Here's how the part is built. I have some questions about the finished solid (model axes, mm). A direction names the side the tool comes from. Round coordinates to 2 decimals unless told otherwise and drop trailing zeros. Write each loop counter-clockwise with the first axis right and the second up, starting at its lowest first coordinate (ties: lowest second). Pieces come first, ordered by that corner, then holes. Notation, with made-up numbers: (-14, 15) -> (27, 15) arc R19 ccw to (27, 21) -> close; hole circle Ø11 at (9, 87.5). An arc over 180 degrees is marked (long way). Answer in a Markdown table with one row per item. Add a question column.
from build123d import *

# Parameters (mm, degrees)
BOSS_EXTRUDE1_DEPTH = 2


with BuildPart() as part:
    # Sketch3 → Boss-Extrude1 (new body)
    with BuildSketch(Plane(origin=(0, 0, 0), x_dir=(0, 0, -1), z_dir=(1, 0, 0))):
        with BuildLine():
            Line((-58.824606693, -2534.80652233), (-1.666930044, -2633.80652233))
            ThreePointArc((-1.666930044, -2633.80652233), (15.902289338, -2651.375741711), (39.902289338, -2657.80652233))
            Line((39.902289338, -2657.80652233), (202.448497275, -2657.80652233))
            ThreePointArc((202.448497275, -2657.80652233), (226.448497275, -2651.375741711), (244.017716657, -2633.80652233))
            Line((244.017716657, -2633.80652233), (301.175393307, -2534.80652233))
            Line((301.175393307, -2534.80652233), (240.287893307, -2534.80652233))
            Line((240.287893307, -2534.80652233), (240.287893307, -2532.80652233))
            Line((240.287893307, -2532.80652233), (216.287893307, -2532.80652233))
            Line((216.287893307, -2532.80652233), (216.287893307, -2534.80652233))
            Line((216.287893307, -2534.80652233), (155.400393307, -2534.80652233))
            Line((155.400393307, -2534.80652233), (155.400393307, -2572.30652233))
            ThreePointArc((155.400393307, -2572.30652233), (153.643033994, -2576.549163017), (149.400393307, -2578.30652233))
            Line((149.400393307, -2578.30652233), (92.950393307, -2578.30652233))
            ThreePointArc((92.950393307, -2578.30652233), (88.70775262, -2576.549163017), (86.950393307, -2572.30652233))
            Line((86.950393307, -2572.30652233), (86.950393307, -2534.80652233))
            Line((86.950393307, -2534.80652233), (43.175393307, -2534.80652233))
            Line((43.175393307, -2534.80652233), (43.175393307, -2532.80652233))
            Line((43.175393307, -2532.80652233), (19.175393307, -2532.80652233))
            Line((19.175393307, -2532.80652233), (19.175393307, -2534.80652233))
            Line((19.175393307, -2534.80652233), (-58.824606693, -2534.80652233))
        make_face()
    extrude(amount=BOSS_EXTRUDE1_DEPTH)


solid = part.part
Item 1: If we section it at C-C on z = -127: Please give me the cut outline in (x, y), then the cut area to 3 significant figures.
Item 2: If we mould it in two halves opening along Z, with no side actions, what happens to faces 3 (the flat face through (0.99, -2583.61, 30.65)), 4 (the cylindrical face through (0.99, -2576.5, -153.69)), 5 (the cylindrical face through (0.986, -2651.551, -226.143))? For each: pulls with the +Z half, pulls with the -Z half, needs draft (parallel to the pull), parting line crosses it, or undercut.
Item 3: I need wall thicknesses on line 1 along Y through (x, z) = (0.7, -187.5); line 2 along Z through (x, y) = (0.9, -2557.5); line 3 along Y through (x, z) = (0.6, -125). Which ranges of each line are inside material? Lowest first, please. Write a range as from..to.
Item 4: If we section it at B-B on x = 1.4: Please give me the cut outline in (y, z), then the cut area to 3 significant figures.
Item 5: If we section it at A-A on y = -2548.5: Please give me the cut outline in (x, z), then the cut area to 3 significant figures.
Item 6: For P1, Ø0.6, axis at x = 1, y = -2533.5, coming from the -Z side; P2, Ø0.6, axis at x = 1, y = -2560, coming from the -Z side; P3, Ø1, axis at x = 0.5, z = -101.5, coming from the +Y side, each with a flat end and sliding along its axis, tell me the tip position at first contact or that it passes through.
Item 7: If we section it at D-D on y = -2596.5: Please give me the cut outline in (x, z).
Item 8: On a 3-axis mill with a long thin cutter (end or side, diameter ignored), from which of +Z, -Z, +X, -X, +Y, -Y can I reach the whole of each face in a straight line? I mean faces 1 (the cylindrical face through (0.986, -2576.596, -88.755)), 2 (the cylindrical face through (1, -2651.2, -15.6)). Say none if no direction works.
Results list:
| question | item | result |
|---|---|---|
| 1 | outline | (0, -2657.81) -> (2, -2657.81) -> (2, -2578.31) -> (0, -2578.31) -> close |
| 1 | area | 159 mm² |
| 2 | face 3 | pulls with the +Z half |
| 2 | face 4 | undercut |
| 2 | face 5 | pulls with the -Z half |
| 3 | line 1 | -2657.81..-2534.81 |
| 3 | line 2 | -288.07..-155.4, -86.95..45.72 |
| 3 | line 3 | -2657.81..-2578.31 |
| 4 | outline | (-2657.81, -202.45) arc R48 ccw to (-2633.81, -244.02) -> (-2534.81, -301.18) -> (-2534.81, -240.29) -> (-2532.81, -240.29) -> (-2532.81, -216.29) -> (-2534.81, -216.29) -> (-2534.81, -155.4) -> (-2572.31, -155.4) arc R6 cw to (-2578.31, -149.4) -> (-2578.31, -92.95) arc R6 cw to (-2572.31, -86.95) -> (-2534.81, -86.95) -> (-2534.81, -43.18) -> (-2532.81, -43.18) -> (-2532.81, -19.18) -> (-2534.81, -19.18) -> (-2534.81, 58.82) -> (-2633.81, 1.67) arc R48 ccw to (-2657.81, -39.9) -> close |
| 4 | area | 32,400 mm² |
| 5 | outline | (0, -293.27) -> (2, -293.27) -> (2, -155.4) -> (0, -155.4) -> close; (0, -86.95) -> (2, -86.95) -> (2, 50.92) -> (0, 50.92) -> close |
| 5 | area | 551 mm² |
| 6 | P1 | z = -240.29 |
| 6 | P2 | z = -286.8 |
| 6 | P3 | y = -2578.31 |
| 7 | outline | (0, -265.56) -> (2, -265.56) -> (2, 23.21) -> (0, 23.21) -> close |
| 8 | face 1 | +X, -X, +Y |
| 8 | face 2 | +Z, +X, -X, -Y |
